from build123d import *

# Parameters (mm, degrees)
F2_W     = 229.145602
F2_H     = 154.409528
F3_DEPTH = 63.5


with BuildPart() as f1:
    # F0 (on Top) → F1 (revolve)
    with BuildSketch(Plane.XY):
        with BuildLine():
            Line((-76.2, 19.05), (-76.2, 0))
            Line((-76.2, 0), (76.2, 0))
            Line((76.2, 0), (76.2, 34.925))
            ThreePointArc((76.2, 34.925), (73.321803, 40.241868), (67.296352, 40.738895))
            Line((67.296352, 40.738895), (52.49993, 34.239835))
            ThreePointArc((52.49993, 34.239835), (44.42729, 31.994194), (36.048919, 32.109551))
            Line((36.048919, 32.109551), (-12.584829, 39.774077))
            ThreePointArc((-12.584829, 39.774077), (-26.724262, 41.172374), (-40.930638, 40.93221))
            ThreePointArc((-40.930638, 40.93221), (-52.695618, 37.488147), (-62.031521, 29.543512))
            ThreePointArc((-62.031521, 29.543512), (-68.382458, 23.306641), (-76.2, 19.05))
        make_face()
    revolve(axis=Axis((0, 0, 0), (1, 0, 0)))

    # F2 (on Top) → F3 (join)
    with BuildSketch(Plane.XY):
        Rectangle(F2_W, F2_H)
    extrude(amount=-F3_DEPTH)


solid = f1.part
Work out the finished part from the listing and answer in its coordinate system (mm). A direction names the side the tool comes from. Coordinates: 2 decimals unless noted, no trailing zeros. Write each loop counter-clockwise with the first axis right and the second up, starting at its lowest first coordinate (ties: lowest second). Pieces come first, ordered by that corner, then holes. Notation, with made-up numbers: (-7, -21) - (46, -21) arc R22 ccw to (46, -12) - close; hole circle Ø5 at (66, 25.5). An arc over 180 degrees is marked (long way). One line per question, with ' | ' between items.
1) Find section B-B, the plane x = 16.5. Determine the outline of the cut face in (y, z).
Checks:
outline: (-77.2, -63.5) - (77.2, -63.5) - (77.2, 0) - (35.19, 0) arc R35.19 ccw to (-35.19, 0) - (-77.2, 0) - close
2) For faces 1 (the face through (24, 35, 0)), 2 (the face through (76.2, 0, 14)), 3 (the face through (-2, 77.205, -31)), determine the directions among +Z, -Z, +X, -X, +Y, -Y from which every point of the face is accessible in a straight line to the end or side of a thin tool.
Checks:
face 1: +Z | face 2: +Z, +X, +Y, -Y | face 3: +Z, -Z, +X, -X, +Y
3) Find section C-C, the plane x = 48. Determine the outline of the cut face in (y, z).
Checks:
outline: (-77.2, -63.5) - (77.2, -63.5) - (77.2, 0) - (32.68, 0) arc R32.68 ccw to (-32.68, 0) - (-77.2, 0) - close
4) Consider probe 1 along Y at (x, z) = (-48.5, 26); probe 2 along Z at (x, y) = (8, -43); probe 3 along X at (y, z) = (22, 18.5). Determine where each line is inside the solid, lowest interval first. Write a range as [from, to].
Checks:
probe 1: [-29.53, 29.53] | probe 2: [-63.5, 0] | probe 3: [-62.67, 76.2]
5) The mould has two halves that part along X. Classify faces 4 (the face through (114.573, -1, -31)), 5 (the face through (-76.2, 0, 8)), 6 (the face through (-2, -77.205, -31)), 7 (the face through (54.86, 0.78, 35.27)): +X half, -X half, draft (parallel to the pull), parting line (faces both ways), or undercut.
Checks:
face 4: +X half | face 5: -X half | face 6: draft | face 7: undercut
6) Flat-ended cylindrical pins translate along their axes: P1, Ø5.5, axis at y = -9.5, z = 13, coming from the -X side; P2, Ø5, axis at x = 6.5, z = 23.5, coming from the -Y side; P3, Ø10.5, axis at y = 6.5, z = 24.5, coming from the +X side. Find the tip coordinate at first contact, or state that the pin passes through.
Checks:
P1: x = -76.2 | P2: y = -30.24 | P3: x = 76.2
7) Find section A-A, the plane y = -44.5. Determine the outline of the cut face in (x, z), and give its area (3 significant figures).
Checks:
outline: (-114.57, -63.5) - (114.57, -63.5) - (114.57, 0) - (-114.57, 0) - close | area: 14,600 mm2
